```python
from build123d import *

# Parameters (mm, degrees)
BOSS_EXTRUDE1_DEPTH = 14.1
CUT_EXTRUDE1_DEPTH  = 14.1
SKETCH3_R           = 2.75
CUT_EXTRUDE2_DEPTH  = 56.302983645


with BuildPart() as part:
    # Sketch1 → Boss-Extrude1 (new body)
    with BuildSketch(Plane.XY):
        Polygon((0, 0), (42, 0), (42, 6.6), (30, 6.6), (30, 33.1), (12, 33.1), (12, 6.6), (0, 6.6), align=None)
    extrude(amount=-BOSS_EXTRUDE1_DEPTH)

    # Sketch2 → Cut-Extrude1 (cut)
    with BuildSketch(Plane.XY):
        with BuildLine():
            Line((20.25, 33.1), (21.75, 33.1))
            Line((21.75, 33.1), (21.75, 23.529058411))
            ThreePointArc((21.75, 23.529058411), (21, 15.6), (20.25, 23.529058411))
            Line((20.25, 23.529058411), (20.25, 33.1))
        make_face()
    extrude(amount=-CUT_EXTRUDE1_DEPTH, mode=Mode.SUBTRACT)

    # Sketch3 → Cut-Extrude2 (cut, through all)
    with BuildSketch(Plane.XZ):
        with Locations(Location((5, -7.05, 0), (0, 0, 270))):
            Circle(SKETCH3_R)
        with Locations(Location((37, -7.05, 0), (0, 0, 270))):
            Circle(SKETCH3_R)
    extrude(amount=-CUT_EXTRUDE2_DEPTH, mode=Mode.SUBTRACT)


solid = part.part
```
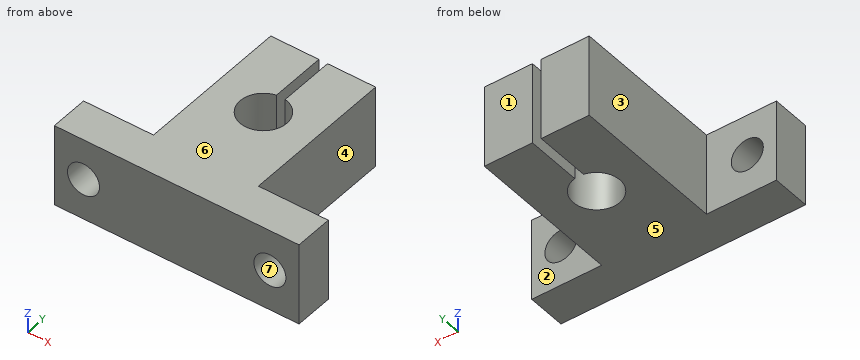
The model under review builds one solid part; all positions refer to its coordinate system, in mm. Face numbers are marked on the shaded views. A direction names the side the tool comes from. Round coordinates to 2 decimals unless told otherwise and drop trailing zeros. Loops run counter-clockwise (first coordinate to the right, second up) from the corner with the lowest first, then second, coordinate; pieces in that order, holes last.
1) Tool access review of the marked faces 1, 2 and 3: name each direction out of +Z, -Z, +X, -X, +Y, -Y from which nothing blocks a thin tool from reaching the whole face with its end or side.
Values follow:
face 1: +Z, -Z, +X, -X, +Y
face 2: +Z, -Z, +X, +Y
face 3: +Z, -Z, -X, +Y
2) Consider section C-C on z = -5.25. State the section outline as (x, y) points, then the cut area to 3 significant figures.
Values follow:
outline: (0, 0) - (2.92, 0) - (2.92, 6.6) - (0, 6.6) - close; (7.08, 0) - (34.92, 0) - (34.92, 6.6) - (30, 6.6) - (30, 33.1) - (21.75, 33.1) - (21.75, 23.53) arc R4 cw (long way) to (20.25, 23.53) - (20.25, 33.1) - (12, 33.1) - (12, 6.6) - (7.08, 6.6) - close; (39.08, 0) - (42, 0) - (42, 6.6) - (39.08, 6.6) - close
area: 635 mm2
3) Consider section D-D on z = -11.5. State the section outline as (x, y) points, then the cut area to 3 significant figures.
Values follow:
outline: (0, 0) - (42, 0) - (42, 6.6) - (30, 6.6) - (30, 33.1) - (21.75, 33.1) - (21.75, 23.53) arc R4 cw (long way) to (20.25, 23.53) - (20.25, 33.1) - (12, 33.1) - (12, 6.6) - (0, 6.6) - close
area: 690 mm2
4) Consider section B-B on y = 30. State the section outline as (x, z) points.
Values follow:
outline: (12, -14.1) - (20.25, -14.1) - (20.25, 0) - (12, 0) - close; (21.75, -14.1) - (30, -14.1) - (30, 0) - (21.75, 0) - close
5) Consider section A-A on x = 37. State the section outline as (y, z) points.
Values follow:
outline: (0, -14.1) - (6.6, -14.1) - (6.6, -9.8) - (0, -9.8) - close; (0, -4.3) - (6.6, -4.3) - (6.6, 0) - (0, 0) - close
6) Wall thickness on line 1 along X through (y, z) = (4.25, -7.05); line 2 along X through (y, z) = (24, -2.25); line 3 along X through (y, z) = (19.6, -7.5): over which ranges is each line inside the solid? List them lowest first.
Values follow:
line 1: x = 0 to 2.25, 7.75 to 34.25, 39.75 to 42
line 2: x = 12 to 20.25, 21.75 to 30
line 3: x = 12 to 17, 25 to 30
7) Clearance check with flat-ended pins moving along their axes: P1, Ø4, axis at y = 16, z = -5, coming from the +X side; P2, Ø7, axis at y = 21, z = -6, coming from the -X side; P3, Ø6, axis at x = 4.5, z = -5.5, coming from the +Y side; P4, Ø5, axis at x = 37, z = -7.05, coming from the +Y side. State where each tip first meets the part, or that it passes through.
Values follow:
P1: stops at x = 30
P2: stops at x = 12
P3: stops at y = 6.6
P4: passes through
8) The part is to be moulded in two halves that separate along Z. For the marked faces 4, 5, 6 and 7, say which applies: pulls with the +Z half, pulls with the -Z half, needs draft (parallel to the pull), parting line crosses it, or undercut.
Values follow:
face 4: needs draft
face 5: pulls with the -Z half
face 6: pulls with the +Z half
face 7: undercut
